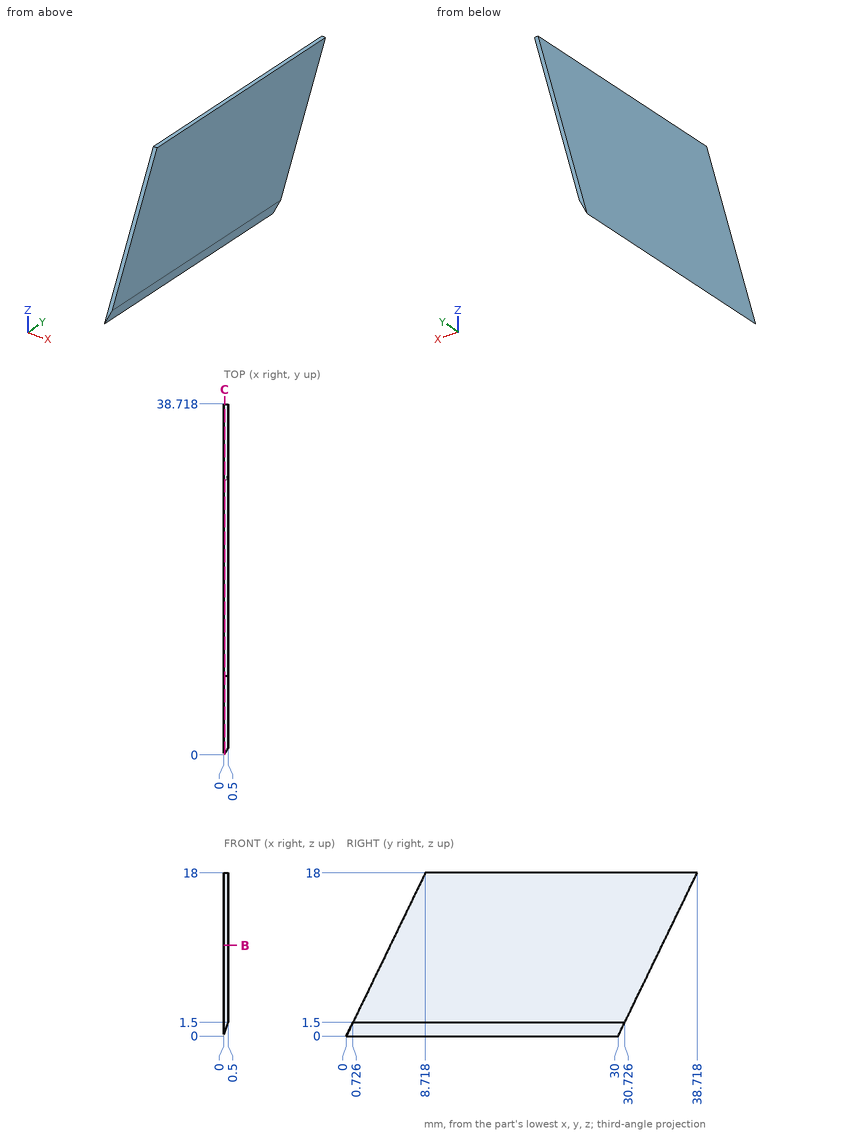
Input: dimensioned drawing with shaded views. Units: mm. Origin: part minimum x, y, z. Round coordinates to 2 decimals unless told otherwise and drop trailing zeros. Loops run counter-clockwise (first coordinate to the right, second up) from the corner with the lowest first, then second, coordinate; pieces in that order, holes last.
1) Section query C-C on x = 0.1. Return the cut outline in (y, z) (1 decimal), plus the area to 3 significant figures.
Ans:
outline: (0.1, 0.3) - (30.1, 0.3) - (38.7, 18) - (8.7, 18) - close
area: 531 mm2
2) Section query B-B on z = 10. Return the cut outline in (x, y).
Ans:
outline: (0, 4.84) - (0.5, 4.84) - (0.5, 34.84) - (0, 34.84) - close
3) Material intervals for line 1 (Y direction, x = 0.2, z = 11.5); line 2 (Y direction, x = 0.2, z = 1.5) (1 decimal); line 3 (Z direction, x = 0.45, y = 33.5) (1 decimal), sorted ascending.
Ans:
line 1: y = 5.57 to 35.57
line 2: y = 0.7 to 30.7
line 3: z = 7.2 to 18
4) Pin query (flat end, axial travel): pin 1 (6 mm diameter, centred on y = 7, z = 13, fed in from -X). Return the tip coordinate at first contact, or that it passes through.
Ans:
pin 1: stops at x = 0
